from build123d import *

# Parameters (mm, degrees)
SKETCH1_W           = 14
SKETCH1_H           = 18.5
SKETCH1_R           = 3.5
SKETCH1_W_2         = 8
SKETCH1_H_2         = 3
BOSS_EXTRUDE1_DEPTH = 6


with BuildPart() as part:
    # Sketch1 → Boss-Extrude1 (new body)
    with BuildSketch(Plane.XY):
        Rectangle(SKETCH1_W, SKETCH1_H)
        with Locations((0, 2.25)):
            Circle(SKETCH1_R, mode=Mode.SUBTRACT)
        with Locations((0, -4.75)):
            Rectangle(SKETCH1_W_2, SKETCH1_H_2, mode=Mode.SUBTRACT)
    extrude(amount=BOSS_EXTRUDE1_DEPTH)


solid = part.part
Build history of the part. All positions in model axes, mm. A direction names the side the tool comes from. Round coordinates to 2 decimals unless told otherwise and drop trailing zeros. Loops run counter-clockwise (first coordinate to the right, second up) from the corner with the lowest first, then second, coordinate; pieces in that order, holes last. Notation, with made-up numbers: (82, 47) -> (132, 47) arc R31 cw to (132, 82) -> close; hole circle Ø6 at (-18.5, 78). An arc over 180 degrees is marked (long way). Answer in a Markdown table with one row per item.
Item 1: Saw through at D-D (x = -3.25). Write the cut outline in (y, z).
Answers below:
| item | result |
|---|---|
| outline | (-9.25, 0) -> (-6.25, 0) -> (-6.25, 6) -> (-9.25, 6) -> close; (-3.25, 0) -> (0.95, 0) -> (0.95, 6) -> (-3.25, 6) -> close; (3.55, 0) -> (9.25, 0) -> (9.25, 6) -> (3.55, 6) -> close |
Item 2: Which spindle directions (+Z, -Z, +X, -X, +Y, -Y) get a long thin tool onto all of the face, cutting with end or side? Do faces 1 (the flat face through (0, -6.25, 3)), 2 (the flat face through (0, -2, 6)). Say none if no direction does.
Answers below:
| item | result |
|---|---|
| face 1 | +Z, -Z |
| face 2 | +Z, +X, -X, +Y, -Y |
Item 3: Mould opens along X. For faces 3 (the flat face through (-7, 0, 3)), 4 (the flat face through (-4, -5, 3)), 5 (the flat face through (0, -9.25, 3)) say: +X half, -X half, draft (parallel to the pull), parting line (faces both ways), or undercut.
Answers below:
| item | result |
|---|---|
| face 3 | -X half |
| face 4 | undercut |
| face 5 | draft |
Item 4: Drill centre lines: L1, parallel to Y at x = 0, z = 1.45; L2, parallel to Y at x = 3.75, z = 1.9; L3, parallel to Y at x = 2.75, z = 1. Where is each one in solid material? Low to high. Write a range as [from, to].
Answers below:
| item | result |
|---|---|
| L1 | y = [-9.25, -6.25], [-3.25, -1.25], [5.75, 9.25] |
| L2 | y = [-9.25, -6.25], [-3.25, 9.25] |
| L3 | y = [-9.25, -6.25], [-3.25, 0.08], [4.42, 9.25] |
Item 5: Saw through at B-B (z = 3.9). Write the cut outline in (x, y), and give its area (3 significant figures).
Answers below:
| item | result |
|---|---|
| outline | (-7, -9.25) -> (7, -9.25) -> (7, 9.25) -> (-7, 9.25) -> close; hole (-4, -6.25) -> (4, -6.25) -> (4, -3.25) -> (-4, -3.25) -> close; hole circle Ø7 at (0, 2.25) |
| area | 197 mm² |
Item 6: Saw through at C-C (y = 2.25). Write the cut outline in (x, z).
Answers below:
| item | result |
|---|---|
| outline | (-7, 0) -> (-3.5, 0) -> (-3.5, 6) -> (-7, 6) -> close; (3.5, 0) -> (7, 0) -> (7, 6) -> (3.5, 6) -> close |
Item 7: Saw through at A-A (x = 0). Write the cut outline in (y, z).
Answers below:
| item | result |
|---|---|
| outline | (-9.25, 0) -> (-6.25, 0) -> (-6.25, 6) -> (-9.25, 6) -> close; (-3.25, 0) -> (-1.25, 0) -> (-1.25, 6) -> (-3.25, 6) -> close; (5.75, 0) -> (9.25, 0) -> (9.25, 6) -> (5.75, 6) -> close |
